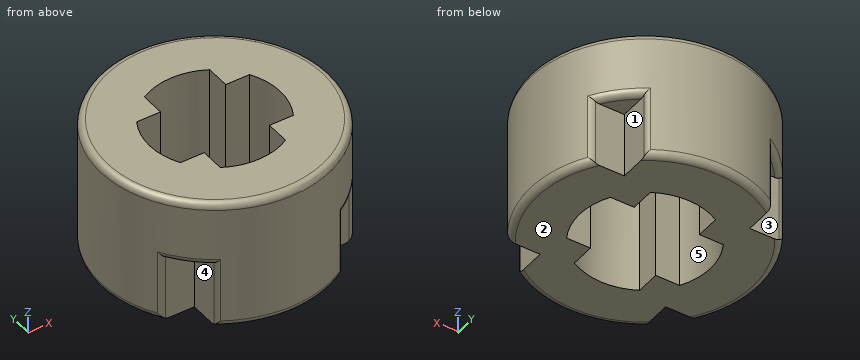
```python
from build123d import *

# Parameters (mm, degrees)
SKETCH1_R           = 3.5
BOSS_EXTRUDE1_DEPTH = 4
SKETCH2_W           = 1
SKETCH2_H           = 1
CUT_EXTRUDE1_DEPTH  = 2
FILLET1_R           = 0.2


with BuildPart() as part:
    # Sketch1 → Boss-Extrude1 (new body)
    with BuildSketch(Plane.XY):
        Circle(SKETCH1_R)
        with BuildLine():
            Line((1, -1), (1.732050808, -1))
            ThreePointArc((1.732050808, -1), (2, 0), (1.732050808, 1))
            Line((1.732050808, 1), (1, 1))
            Line((1, 1), (1, 1.732050808))
            ThreePointArc((1, 1.732050808), (0, 2), (-1, 1.732050808))
            Line((-1, 1.732050808), (-1, 1))
            Line((-1, 1), (-1.732050808, 1))
            ThreePointArc((-1.732050808, 1), (-2, 0), (-1.732050808, -1))
            Line((-1.732050808, -1), (-1, -1))
            Line((-1, -1), (-1, -1.732050808))
            ThreePointArc((-1, -1.732050808), (0, -2), (1, -1.732050808))
            Line((1, -1.732050808), (1, -1))
        make_face(mode=Mode.SUBTRACT)
    extrude(amount=BOSS_EXTRUDE1_DEPTH)

    # Sketch2 → Cut-Extrude1 (cut)
    with BuildSketch(Plane(origin=(0, 0, 0), x_dir=(-1, 0, 0), z_dir=(0, 0, -1))):
        with Locations((-2.423839929, 2.423839929)):
            Rectangle(SKETCH2_W, SKETCH2_H)
        with Locations((-2.423839929, -2.423839929)):
            Rectangle(SKETCH2_W, SKETCH2_H)
        with Locations((2.423839929, -2.423839929)):
            Rectangle(SKETCH2_W, SKETCH2_H)
        with Locations((2.423839929, 2.423839929)):
            Rectangle(SKETCH2_W, SKETCH2_H)
    extrude(amount=-CUT_EXTRUDE1_DEPTH, mode=Mode.SUBTRACT)

    # Fillet1
    fillet1_edges = [part.edges().sort_by_distance(p)[0] for p in [
        (0, 3.5, 0),
        (-3.5, 0, 0),
        (0, -3.5, 0),
        (3.352867411, 1.004131528, 0),
        (2.474873734, 2.474873734, 2),
        (2.474873734, -2.474873734, 2),
        (-3.5, 0, 4),
        (-2.474873734, -2.474873734, 2),
        (-2.474873734, 2.474873734, 2),
        (-2.923839929, 1.923839929, 1),
        (-1.923839929, 2.923839929, 1),
        (-1.923839929, -2.923839929, 1),
        (-2.923839929, -1.923839929, 1),
        (2.923839929, -1.923839929, 1),
        (1.923839929, -2.923839929, 1),
        (2.923839929, 1.923839929, 1),
        (1.923839929, 2.923839929, 1),
    ]]
    fillet(fillet1_edges, radius=FILLET1_R)


solid = part.part
```
Input: part model. Units: mm. Frame: model coordinates. Face numbers are marked on the shaded views. A direction names the side the tool comes from. Coordinates: 2 decimals unless noted, no trailing zeros. Write each loop counter-clockwise with the first axis right and the second up, starting at its lowest first coordinate (ties: lowest second). Pieces come first, ordered by that corner, then holes.
1) Material intervals for line 1 along Y through (x, z) = (1.5, 1.55); line 2 along X through (y, z) = (0.75, 1.15); line 3 along X through (y, z) = (-0.25, 3.25), sorted ascending.
2) Section B-B on x = 0. Output: boundary loops of the cut face in (y, z), and give its area (3 significant figures).
3) Set-up query: the marked faces 1, 2, 3, 4 and 5. Return all of +Z, -Z, +X, -X, +Y, -Y with unobstructed straight access to the full face (end or side cutting, diameter ignored); none if empty.
4) Pin query (flat end, axial travel): pin 1 Ø1 at (x, z) = (-2, 1) entering from -Y; pin 2 Ø1 at (x, z) = (2.5, 0.5) entering from +Y; pin 3 Ø0.7 at (y, z) = (2, 1) entering from +X. Return the tip coordinate at first contact, or that it passes through.
Check result:
1. line 1: y = -3.16 to -1, 1 to 3.16
1. line 2: x = -3.42 to -1.85, 1.85 to 3.42
1. line 3: x = -3.49 to -1.98, 1.98 to 3.49
2. outline: (-3.5, 0.2) arc R0.2 ccw to (-3.3, 0) - (-2, 0) - (-2, 4) - (-3.3, 4) arc R0.2 ccw to (-3.5, 3.8) - close; (2, 0) - (3.3, 0) arc R0.2 ccw to (3.5, 0.2) - (3.5, 3.8) arc R0.2 ccw to (3.3, 4) - (2, 4) - close
2. area: 12.0 mm2
3. face 1: -Z, +X, +Y
3. face 2: -Z, +X, -X, +Y, -Y
3. face 3: -Z, -X, +Y
3. face 4: -Z, -X, -Y
3. face 5: +Z, -Z
4. pin 1: stops at y = -3.16
4. pin 2: stops at y = 1.92
4. pin 3: stops at x = 3.09
